Source: CAD feature listing. Evaluate the final solid. Frame: model axes, mm. Coordinates: 2 decimals unless noted, no trailing zeros. Order: outer loops, then holes, each group sorted by start corner. A loop starts at its lowest first (then second) coordinate and runs counter-clockwise, first axis right, second up. Notation, with made-up numbers: (-38.75, 72) - (-30.75, 72) arc R5 ccw to (-30.75, 81) - close; hole circle Ø10 at (59, -0.75). An arc over 180 degrees is marked (long way). One line per question, with ' | ' between items. Start each with the question number.
(1) Line query: line 1 along Y through (x, z) = (48.5, 25.4); line 2 along Z through (x, y) = (-46, 0). Output: solid intervals per line, ascending.
(2) Section C-C (x = 37). Return the cut outline in (y, z), then the cut area to 3 significant figures.
(3) Section B-B (y = -8). Return the cut outline in (x, z).
(4) Section A-A (z = 25.4). Return the cut outline in (x, y), then the cut area to 3 significant figures.
(5) Contact query for a flat-ended pin moving along its axis: P1, Ø15, axis at y = 0, z = 25.4, coming from the +X side. Output: stop coordinate, or through.
(6) Draft query along X for faces 1 (the flat face through (76.2, 16, 25)), 2 (the flat face through (16, 76.2, 25)), 3 (the flat face through (-76.2, 16, 25)), 4 (the cylindrical face through (-12.114, -37.567, 29.215)). Return one class per face: +X half, -X half, draft (parallel to the pull), parting line (faces both ways), or undercut.
from build123d import *

# Parameters (mm, degrees)
F0_W     = 152.4
F0_H     = 152.4
F1_DEPTH = 50.8
F3_R     = 12.7
F4_DEPTH = 152.4
F2_R     = 12.7
F5_DEPTH = 152.4


with BuildPart() as f1:
    # F0 (on Top) → F1 (new body)
    with BuildSketch(Plane.XY):
        Rectangle(F0_W, F0_H)
    extrude(amount=F1_DEPTH)

    # F3 (on face) → F4 (cut)
    with BuildSketch(Plane(origin=(0, 76.2, 0), x_dir=(-1, 0, 0), z_dir=(0, 1, 0))):
        with Locations((0, 25.4)):
            Circle(F3_R)
    extrude(amount=-F4_DEPTH, mode=Mode.SUBTRACT)

    # F2 (on face) → F5 (cut)
    with BuildSketch(Plane(origin=(-76.2, 0, 0), x_dir=(0, -1, 0), z_dir=(-1, 0, 0))):
        with Locations((0, 25.4)):
            Circle(F2_R)
    extrude(amount=-F5_DEPTH, mode=Mode.SUBTRACT)


solid = f1.part
Response values:
1) line 1: y = -76.2 to -12.7, 12.7 to 76.2 | line 2: z = 0 to 12.7, 38.1 to 50.8
2) outline: (-76.2, 0) - (76.2, 0) - (76.2, 50.8) - (-76.2, 50.8) - close; hole circle Ø25.4 at (0, 25.4) | area: 7,240 mm²
3) outline: (-76.2, 0) - (76.2, 0) - (76.2, 15.54) - (8, 15.54) arc R12.7 cw to (-8, 15.54) - (-76.2, 15.54) - close; (-76.2, 35.26) - (-8, 35.26) arc R12.7 cw to (8, 35.26) - (76.2, 35.26) - (76.2, 50.8) - (-76.2, 50.8) - close
4) outline: (-76.2, -76.2) - (-12.7, -76.2) - (-12.7, -12.7) - (-76.2, -12.7) - close; (-76.2, 12.7) - (-12.7, 12.7) - (-12.7, 76.2) - (-76.2, 76.2) - close; (12.7, -76.2) - (76.2, -76.2) - (76.2, -12.7) - (12.7, -12.7) - close; (12.7, 12.7) - (76.2, 12.7) - (76.2, 76.2) - (12.7, 76.2) - close | area: 16,100 mm²
5) P1: passes through
6) face 1: +X half | face 2: draft | face 3: -X half | face 4: undercut
